Source: CAD feature listing. Evaluate the final solid. Frame: model axes, mm. A direction names the side the tool comes from. Round coordinates to 2 decimals unless told otherwise and drop trailing zeros. Write each loop counter-clockwise with the first axis right and the second up, starting at its lowest first coordinate (ties: lowest second). Pieces come first, ordered by that corner, then holes. Notation, with made-up numbers: M -10,53.25 L -6,53.25 A5 ccw -6,60.25 Z; hole C 80.25,-10 d2. An arc over 180 degrees is marked long. Use a Markdown table: item, result.
```python
from build123d import *

# Parameters (mm, degrees)
F0_W     = 40
F0_H     = 40
F1_DEPTH = 20
F2_W     = 10
F2_H     = 10
F3_DEPTH = 10
F4_W     = 10
F4_H     = 10
F5_DEPTH = 10


with BuildPart() as f1:
    # F0 (on Front) → F1 (new body, symmetric)
    with BuildSketch(Plane.XZ):
        Rectangle(F0_W, F0_H)
    extrude(amount=F1_DEPTH, both=True)

    # F2 (on face) → F3 (join)
    with BuildSketch(Plane.XZ.offset(20)):
        Rectangle(F2_W, F2_H)
    extrude(amount=F3_DEPTH)

    # F4 (on face) → F5 (join)
    with BuildSketch(Plane(origin=(-20, 0, 0), x_dir=(0, -1, 0), z_dir=(-1, 0, 0))):
        Rectangle(F4_W, F4_H)
    extrude(amount=F5_DEPTH)


solid = f1.part
```
Q1. Line query: L1, parallel to Y at x = 17, z = -2.5; L2, parallel to Y at x = -22, z = -1.5. Output: solid intervals per line, ascending.
Results are:
| item | result |
|---|---|
| L1 | -20 to 20 |
| L2 | -5 to 5 |
Q2. Reachability of faces 1 (the flat face through (-25, -5, 0)), 2 (the flat face through (0, -25, 5)), 3 (the flat face through (5, -25, 0)), 4 (the flat face through (-25, 0, -5)) from +Z, -Z, +X, -X, +Y, -Y: full face, straight path, thin tool, end or side. Return the list, or none.
Results are:
| item | result |
|---|---|
| face 1 | +Z, -Z, -X, -Y |
| face 2 | +Z, +X, -X, -Y |
| face 3 | +Z, -Z, +X, -Y |
| face 4 | -Z, -X, +Y, -Y |
Q3. Section A-A on x = 0. Return loops of the section in (y, z).
Results are:
| item | result |
|---|---|
| outline | M -30,-5 L -20,-5 L -20,-20 L 20,-20 L 20,20 L -20,20 L -20,5 L -30,5 Z |
Q4. Section D-D on x = -25.5. Return loops of the section in (y, z).
Results are:
| item | result |
|---|---|
| outline | M -5,-5 L 5,-5 L 5,5 L -5,5 Z |
Q5. Section B-B on z = 3. Return loops of the section in (x, y).
Results are:
| item | result |
|---|---|
| outline | M -30,-5 L -20,-5 L -20,-20 L -5,-20 L -5,-30 L 5,-30 L 5,-20 L 20,-20 L 20,20 L -20,20 L -20,5 L -30,5 Z |
Q6. First-contact query: pin 1 Ø3 at (x, y) = (-23.5, 0) entering from -Z; pin 2 Ø8 at (x, z) = (-22.5, -0.5) entering from -Y; pin 3 Ø1 at (y, z) = (10, 12) entering from -X. Flat tips, straight axial feed; report the tip coordinate or a pass-through.
Results are:
| item | result |
|---|---|
| pin 1 | z = -5 |
| pin 2 | y = -20 |
| pin 3 | x = -20 |
